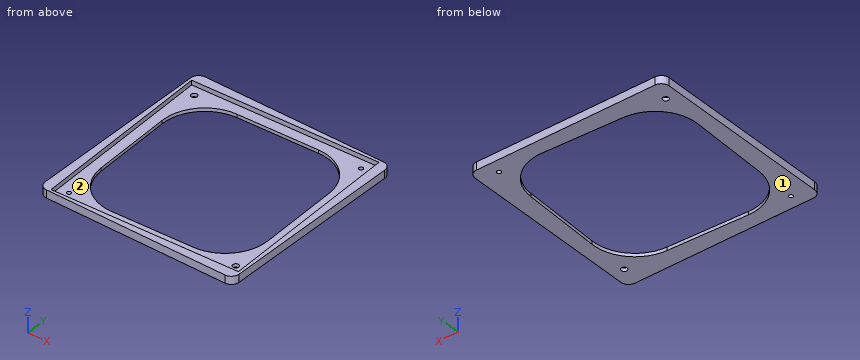
Autodesk Inventor part; units mm, degrees
ref_plane "YZ Plane" through (0, 0, 0) normal (1, 0, 0) x (0, 1, 0)
ref_plane "XZ Plane" through (0, 0, 0) normal (0, 1, 0) x (-1, 0, 0)
ref_plane "XY Plane" through (0, 0, 0) normal (0, 0, 1) x (1, 0, 0)
sketch "スケッチ1" plane through (0, 0, 0) normal (0, 0, 1) x (1, 0, 0)
  line L0 (-75, -215) -> (75, -215)
  line L1 (75, -215) -> (75, 215)
  line L2 (75, 215) -> (-75, 215)
  line L3 (-75, 215) -> (-75, -215)
  line L4 (-75, -215) -> (75, 215) construction
  line L5 (75, -215) -> (-75, 215) construction
  line L6 (-65, -215) -> (-65, 215) construction
  line L7 (-65, 59.8957) -> (59.8957, 65) construction
  line L8 (59.8957, 65) -> (65, -59.8957) construction
  line L9 (65, -59.8957) -> (-59.8957, -65) construction
  line L10 (-59.8957, -65) -> (-65, 59.8957) construction
  line L11 (-65, 59.8957) -> (65, -59.8957) construction
  line L12 (59.8957, 65) -> (-59.8957, -65) construction
  circle A0 centre (-65, 59.8957) radius 2.25
  line L13 (-67.0832, -72.8) -> (72.8, -67.0832) construction
  line L14 (72.8, -67.0832) -> (67.0832, 72.8) construction
  line L15 (67.0832, 72.8) -> (-72.8, 67.0832) construction
  line L16 (-72.8, 67.0832) -> (-67.0832, -72.8) construction
  line L17 (-67.0832, -72.8) -> (67.0832, 72.8) construction
  line L18 (72.8, -67.0832) -> (-72.8, 67.0832) construction
  line L19 (0, 0) -> (0, 70.0584) construction
  circle A1 centre (65, -59.8957) radius 2.25
  circle A2 centre (59.8957, 65) radius 1.6
  circle A3 centre (-59.8957, -65) radius 1.6
  line L20 (-63.6933, 27.9224) -> (-61.2024, -33.0267)
  line L21 (-27.9224, -63.6933) -> (33.0267, -61.2024)
  line L22 (63.6933, -27.9224) -> (61.2024, 33.0267)
  line L23 (27.9224, 63.6933) -> (-33.0267, 61.2024)
  line L24 (-62.4479, -2.5521) -> (62.4479, 2.5521) construction
  arc A4 (-33.0267, 61.2024) -> (-63.6933, 27.9224) centre (-31.72, 29.2291) ccw
  arc A5 (61.2024, 33.0267) -> (27.9224, 63.6933) centre (29.2291, 31.72) ccw
  arc A6 (33.0267, -61.2024) -> (63.6933, -27.9224) centre (31.72, -29.2291) ccw
  arc A7 (-61.2024, -33.0267) -> (-27.9224, -63.6933) centre (-29.2291, -31.72) ccw
  circle A8 centre (-65, -81.1043) radius 2.25
  circle A9 centre (-59.8957, -206) radius 1.6
  circle A10 centre (65, -200.8957) radius 2.25
  circle A11 centre (59.8957, -76) radius 1.6
  arc A12 (61.2024, -107.9733) -> (27.9224, -77.3067) centre (29.2291, -109.28) ccw
  line L25 (27.9224, -77.3067) -> (-33.0267, -79.7976)
  arc A13 (-33.0267, -79.7976) -> (-63.6933, -113.0776) centre (-31.72, -111.7709) ccw
  line L26 (-63.6933, -113.0776) -> (-61.2024, -174.0267)
  arc A14 (-61.2024, -174.0267) -> (-27.9224, -204.6933) centre (-29.2291, -172.72) ccw
  line L27 (-27.9224, -204.6933) -> (33.0267, -202.2024)
  arc A15 (33.0267, -202.2024) -> (63.6933, -168.9224) centre (31.72, -170.2291) ccw
  line L28 (63.6933, -168.9224) -> (61.2024, -107.9733)
  circle A16 centre (-65, 200.8957) radius 2.25
  circle A17 centre (-59.8957, 76) radius 1.6
  circle A18 centre (65, 81.1043) radius 2.25
  circle A19 centre (59.8957, 206) radius 1.6
  arc A20 (61.2024, 174.0267) -> (27.9224, 204.6933) centre (29.2291, 172.72) ccw
  line L29 (27.9224, 204.6933) -> (-33.0267, 202.2024)
  arc A21 (-33.0267, 202.2024) -> (-63.6933, 168.9224) centre (-31.72, 170.2291) ccw
  line L30 (-63.6933, 168.9224) -> (-61.2024, 107.9733)
  arc A22 (-61.2024, 107.9733) -> (-27.9224, 77.3067) centre (-29.2291, 109.28) ccw
  line L31 (-27.9224, 77.3067) -> (33.0267, 79.7976)
  arc A23 (33.0267, 79.7976) -> (63.6933, 113.0776) centre (31.72, 111.7709) ccw
  line L32 (63.6933, 113.0776) -> (61.2024, 174.0267)
  circle A24 centre (-65, 59.8957) radius 2.25
  circle A25 centre (-59.8957, -65) radius 1.6
  circle A26 centre (65, -59.8957) radius 2.25
  circle A27 centre (59.8957, 65) radius 1.6
  arc A28 (61.2024, 33.0267) -> (27.9224, 63.6933) centre (29.2291, 31.72) ccw
  line L33 (27.9224, 63.6933) -> (-33.0267, 61.2024)
  arc A29 (-33.0267, 61.2024) -> (-63.6933, 27.9224) centre (-31.72, 29.2291) ccw
  line L34 (-63.6933, 27.9224) -> (-61.2024, -33.0267)
  arc A30 (-61.2024, -33.0267) -> (-27.9224, -63.6933) centre (-29.2291, -31.72) ccw
  line L35 (-27.9224, -63.6933) -> (33.0267, -61.2024)
  arc A31 (33.0267, -61.2024) -> (63.6933, -27.9224) centre (31.72, -29.2291) ccw
  line L36 (63.6933, -27.9224) -> (61.2024, 33.0267)
  point P0 (-65, 59.8957)
  point P1 (59.8957, 65)
  point P2 (-65, -81.1043)
  point P3 (59.8957, -76)
  point P4 (-62.4479, -143.5521)
  point P5 (62.4479, -138.4479)
  point P6 (-65, 200.8957)
  point P7 (59.8957, 206)
  point P8 (-62.4479, 138.4479)
  point P9 (62.4479, 143.5521)
  point P10 (-65, 59.8957)
  point P11 (59.8957, 65)
  dimension "d0" = 150
  dimension "d1" = 430
  dimension "d3" = 65
  dimension "d4" = 125
  dimension "d7" = 4.5
  dimension "d8" = 140
  dimension "d9" = 70.0584
  dimension "d10" = 3.2
  dimension "d24" = 125
  dimension "d25" = 32
  dimension "d28" = 141
  dimension "d31" = 141
extrude "押し出し1" add sketch "スケッチ1" along normal blind 6 contours L3 L2 L1 L0 | A8 | A11 | A17 | A18
sketch "スケッチ4" plane through (0, 0, 6) normal (0, 0, 1) x (1, 0, 0)
  line L0 (-75, 75) -> (75, 75)
  line L1 (75, 75) -> (75, -75)
  line L2 (75, -75) -> (-75, -75)
  line L3 (-75, -75) -> (-75, 75)
  point P0 (0, 0)
  point P1 (-75, 0)
  point P2 (0, 75)
  dimension "d43" = 150
  dimension "d46" = 150
extrude "押し出し3" cut sketch "スケッチ4" against normal through all keep common part
sketch "スケッチ5" plane through (0, 0, 6) normal (0, 0, 1) x (1, 0, 0)
  line L0 (-73.008, 67.2749) -> (-67.2749, -73.008)
  line L1 (-67.2749, -73.008) -> (73.008, -67.2749)
  line L2 (73.008, -67.2749) -> (67.2749, 73.008)
  line L3 (67.2749, 73.008) -> (-73.008, 67.2749)
  line L4 (-33.0267, 61.2024) -> (27.9224, 63.6933) construction
  line L5 (67.2749, 73.008) -> (-67.2749, -73.008) construction
  point P0 (0, 0)
  point P1 (0, 0)
  dimension "d47" = 140.4
extrude "押し出し4" cut sketch "スケッチ5" against normal blind 3.5
fillet "フィレット2" radius 6 4 edges at (-75, 75, 3) (-75, -75, 3) (75, -75, 3) (75, 75, 3)
properties part number "bottom_140mm" material "アルミニウム 6061"
Geometry: final body of the model. Coordinates: model frame, mm. Face numbers are marked on the shaded views. Coordinates: 2 decimals unless noted, no trailing zeros. Order: outer loops, then holes, each group sorted by start corner. A loop starts at its lowest first (then second) coordinate and runs counter-clockwise, first axis right, second up.
1) Section A-A (z = 4). Return loops of the section in (x, y), then the cut area to 3 significant figures.
Result sheet:
outline: (-75, -69) arc R6 ccw to (-69, -75) - (69, -75) arc R6 ccw to (75, -69) - (75, 69) arc R6 ccw to (69, 75) - (-69, 75) arc R6 ccw to (-75, 69) - close; hole (-73.01, 67.27) - (-67.27, -73.01) - (73.01, -67.27) - (67.27, 73.01) - close
area: 2,760 mm2
2) Section C-C (x = -39.5). Return loops of the section in (y, z), then the cut area to 3 significant figures.
Result sheet:
outline: (-75, 0) - (-62.03, 0) - (-62.03, 2.5) - (-71.87, 2.5) - (-71.87, 6) - (-75, 6) - close; (60.27, 0) - (75, 0) - (75, 6) - (68.64, 6) - (68.64, 2.5) - (60.27, 2.5) - close
area: 102 mm2
3) First-contact query: P1, Ø2.5, axis at x = -59.9, y = -65, coming from the -Z side; P2, Ø5, axis at x = 59.9, y = 65, coming from the +Z side. Flat tips, straight axial feed; report the tip coordinate or a pass-through.
Result sheet:
P1: passes through
P2: stops at z = 2.5
4) Draft query along Y for the marked faces 1 and 2. Return one class per face: released by +Y, released by -Y, zero draft, split by the parting line, or undercut.
Result sheet:
face 1: zero draft
face 2: undercut
5) Section B-B (y = 21). Return loops of the section in (x, z), then the cut area to 3 significant figures.
Result sheet:
outline: (-75, 0) - (-63.41, 0) - (-63.41, 2.5) - (-71.12, 2.5) - (-71.12, 6) - (-75, 6) - close; (61.69, 0) - (75, 0) - (75, 6) - (69.4, 6) - (69.4, 2.5) - (61.69, 2.5) - close
area: 95.4 mm2
6) Ray query, probe 1 along X at (y, z) = (65, 1.3); probe 2 along X at (y, z) = (-65, 1.35); probe 3 along Y at (x, z) = (65, 0.55). Return the intervals inside material, ascending.
Result sheet:
probe 1: x = -75 to 58.3, 61.5 to 75
probe 2: x = -75 to -61.5, -58.3 to 75
probe 3: y = -75 to -62.15, -57.65 to 75
